Geometry check sheet. Reference: the model listing, model coordinates, mm. Face numbers are marked on the shaded views. A direction names the side the tool comes from. Give positions to 0.01 mm unless a question says otherwise; leave off trailing zeros. Write each loop counter-clockwise with the first axis right and the second up, starting at its lowest first coordinate (ties: lowest second). Pieces come first, ordered by that corner, then holes. Notation, with made-up numbers: (37, 33) - (54, 33) arc R6 ccw to (54, 40) - close; hole circle Ø5 at (43.5, -18). An arc over 180 degrees is marked (long way). Use a Markdown table: item, result.
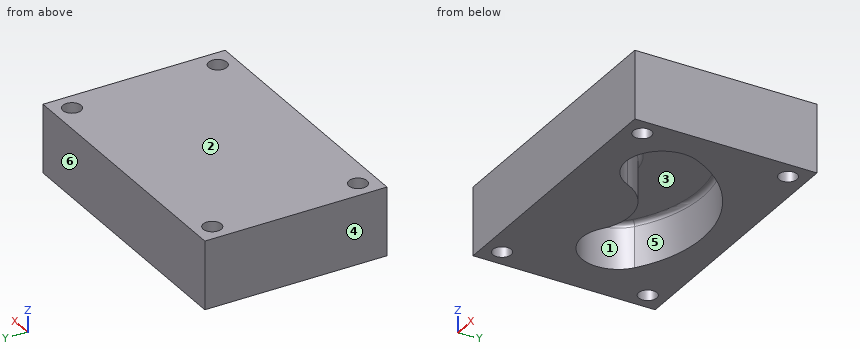
```python
from build123d import *

# Parameters (mm, degrees)
ESQUISSE1_W             = 60
ESQUISSE1_H             = 40
BOSS_EXTRU_1_DEPTH      = 15
ESQUISSE3_R             = 2
ENL_V_MAT_EXTRU_1_DEPTH = 25
ENL_V_MAT_EXTRU_2_DEPTH = 10
CONG_1_R                = 1


with BuildPart() as part:
    # Esquisse1 → Boss.-Extru.1 (new body)
    with BuildSketch(Plane.XY):
        Rectangle(ESQUISSE1_W, ESQUISSE1_H)
    extrude(amount=BOSS_EXTRU_1_DEPTH)

    # Esquisse3 → Enlèv. mat.-Extru.1 (cut)
    with BuildSketch(Plane(origin=(0, 0, 0), x_dir=(-1, 0, 0), z_dir=(0, 0, -1))):
        with Locations((-26, 16)):
            Circle(ESQUISSE3_R)
        with Locations((26, 16)):
            Circle(ESQUISSE3_R)
        with Locations((-26, -16)):
            Circle(ESQUISSE3_R)
        with Locations((26, -16)):
            Circle(ESQUISSE3_R)
    extrude(amount=-ENL_V_MAT_EXTRU_1_DEPTH, mode=Mode.SUBTRACT)

    # Esquisse4 → Enlèv. mat.-Extru.2 (cut)
    with BuildSketch(Plane(origin=(0, 0, 0), x_dir=(-1, 0, 0), z_dir=(0, 0, -1))):
        with BuildLine():
            ThreePointArc((18.333200892, 8.584679084), (-4.652870853, 13.070183937), (-22.581024868, -1.998344249))
            ThreePointArc((-22.581024868, -1.998344249), (-18.601997418, -12.58925264), (-8.011089026, -8.61022519))
            ThreePointArc((-8.011089026, -8.61022519), (-0.646121832, -2.420005289), (8.796660967, -4.26267108))
            ThreePointArc((8.796660967, -4.26267108), (19.988606012, -2.607265961), (18.333200892, 8.584679084))
        make_face()
    extrude(amount=-ENL_V_MAT_EXTRU_2_DEPTH, mode=Mode.SUBTRACT)

    # Congé1
    cong_1_edges = [part.edges().sort_by_distance(p)[0] for p in [
        (-19.988606012, -2.607265961, 10),
        (0.646121832, -2.420005289, 10),
        (18.601997418, -12.58925264, 10),
        (4.652870853, 13.070183937, 10),
    ]]
    fillet(cong_1_edges, radius=CONG_1_R)


solid = part.part
```
1) Section check C-C on z = 11.75. Record the boundary of the cut face in (x, y), then the cut area to 3 significant figures.
Working result:
| item | result |
|---|---|
| outline | (-30, -20) - (30, -20) - (30, 20) - (-30, 20) - close; hole circle Ø4 at (-26, -16); hole circle Ø4 at (-26, 16); hole circle Ø4 at (26, -16); hole circle Ø4 at (26, 16) |
| area | 2,350 mm² |
2) Section check B-B on y = -16. Record the boundary of the cut face in (x, z), then the cut area to 3 significant figures.
Working result:
| item | result |
|---|---|
| outline | (-30, 0) - (-28, 0) - (-28, 15) - (-30, 15) - close; (-24, 0) - (24, 0) - (24, 15) - (-24, 15) - close; (28, 0) - (30, 0) - (30, 15) - (28, 15) - close |
| area | 780 mm² |
3) Section check D-D on z = 6.5. Record the boundary of the cut face in (x, y), then the cut area to 3 significant figures.
Working result:
| item | result |
|---|---|
| outline | (-30, -20) - (30, -20) - (30, 20) - (-30, 20) - close; hole circle Ø4 at (-26, -16); hole circle Ø4 at (-26, 16); hole (-18.33, 8.58) arc R8 ccw to (-8.8, -4.26) arc R11.16 cw to (8.01, -8.61) arc R8 ccw to (22.58, -2) arc R27.16 ccw to start; hole circle Ø4 at (26, -16); hole circle Ø4 at (26, 16) |
| area | 1,600 mm² |
4) Set-up check for the marked faces 1 and 2: record each of +Z, -Z, +X, -X, +Y, -Y from which the full face is reachable in a straight line by a thin tool's end or side.
Working result:
| item | result |
|---|---|
| face 1 | -Z |
| face 2 | +Z, +X, -X, +Y, -Y |
5) Depth check by flat-ended pin: P1, Ø3.5, axis at x = -26, y = -16, coming from the -Z side. Enter the tip coordinate at first touch or a pass-through.
Working result:
| item | result |
|---|---|
| P1 | passes through |
6) Section check A-A on x = -26. Record the boundary of the cut face in (y, z), then the cut area to 3 significant figures.
Working result:
| item | result |
|---|---|
| outline | (-20, 0) - (-18, 0) - (-18, 15) - (-20, 15) - close; (-14, 0) - (14, 0) - (14, 15) - (-14, 15) - close; (18, 0) - (20, 0) - (20, 15) - (18, 15) - close |
| area | 480 mm² |
7) Mould release check, pull along X, two halves, no side actions. Record for the marked faces 3, 4, 5 and 6: pulls with the +X half, pulls with the -X half, needs draft (parallel to the pull), parting line crosses it, or undercut.
Working result:
| item | result |
|---|---|
| face 3 | undercut |
| face 4 | pulls with the -X half |
| face 5 | undercut |
| face 6 | needs draft |
8) Material ranges on L1, parallel to Y at x = 26, z = 7.75; L2, parallel to X at y = -4, z = 7.5; L3, parallel to Z at x = 21, y = -5.5, recorded low to high. Write a range as from..to.
Working result:
| item | result |
|---|---|
| L1 | y = -20..-18, -14..14, 18..20 |
| L2 | x = -30..-18.67, -8.43..4.13, 23.19..30 |
| L3 | z = 10..15 |
